Answer from the drawing. Dimensions are ordinates in mm from the lowest x, y and z of the part. Coordinates: 2 decimals unless noted, no trailing zeros. Write each loop counter-clockwise with the first axis right and the second up, starting at its lowest first coordinate (ties: lowest second). Pieces come first, ordered by that corner, then holes.
(1) The part is cut by section A-A, the plane z = 5.08. Determine the outline of the cut face in (x, y) (3 decimals), and give its area (3 significant figures).
(2) Determine the mould class of the marked faces 1, 2 and 3 for opening direction X: pulls with the +X half, pulls with the -X half, needs draft (parallel to the pull), parting line crosses it, or undercut.
(3) Straight lines are drawn through the part: line 1 along X through (y, z) = (5.25, 8.5); line 2 along Z through (x, y) = (63, 4.75); line 3 along Z through (x, y) = (29, 4.25). For each, find the intervals that lie inside material, in ascending order.
(4) Given pin 1 (3 mm diameter, centred on x = 67.5, z = 7.5, fed in from -Y); pin 2 (1.5 mm diameter, centred on x = 26.5, y = 8, fed in from +Z); pin 3 (2 mm diameter, centred on x = 14, y = 8, fed in from +Z); pin 4 (4 mm diameter, centred on y = 6, z = 8.5, fed in from -X), each flat-ended and moving along its own axis, determine where each tip first touches the part or whether it passes through.
(5) The part is cut by section C-C, the plane x = 27. Determine the outline of the cut face in (y, z) (3 decimals), and give its area (3 significant figures).
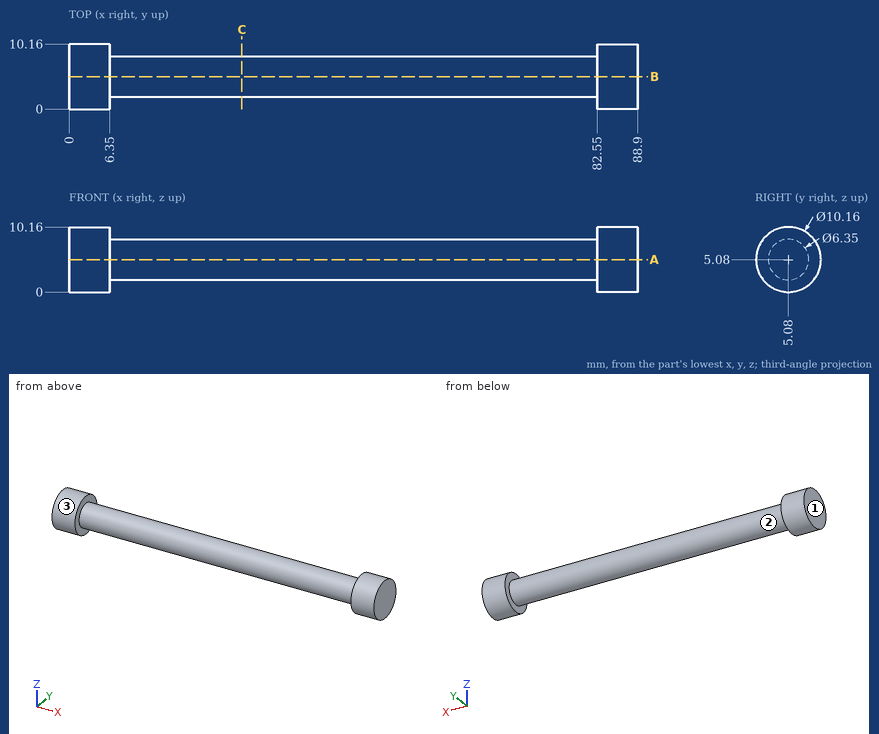
Computed:
1. outline: (0, 0) - (6.35, 0) - (6.35, 1.905) - (82.55, 1.905) - (82.55, 0) - (88.9, 0) - (88.9, 10.16) - (82.55, 10.16) - (82.55, 8.255) - (6.35, 8.255) - (6.35, 10.16) - (0, 10.16) - close
1. area: 613 mm2
2. face 1: pulls with the -X half
2. face 2: undercut
2. face 3: needs draft
3. line 1: x = 0 to 6.35, 82.55 to 88.9
3. line 2: z = 1.92 to 8.24
3. line 3: z = 2.02 to 8.14
4. pin 1: stops at y = 2.04
4. pin 2: stops at z = 7.4
4. pin 3: stops at z = 7.61
4. pin 4: stops at x = 0
5. outline: circle Ø6.35 at (5.08, 5.08)
5. area: 31.7 mm2
